Design review of the part shown in the three views and the two pictorial views. Dimensions are in mm from the part's minimum x, y and z. A direction names the side the tool comes from. Coordinates: 2 decimals unless noted, no trailing zeros. Loops run counter-clockwise (first coordinate to the right, second up) from the corner with the lowest first, then second, coordinate; pieces in that order, holes last. Notation, with made-up numbers: M 12.5,40 L 32.5,40 A28 ccw 32.5,79 Z; hole C 44,-20 d7. An arc over 180 degrees is marked long. Use one line per item in the form item = value.
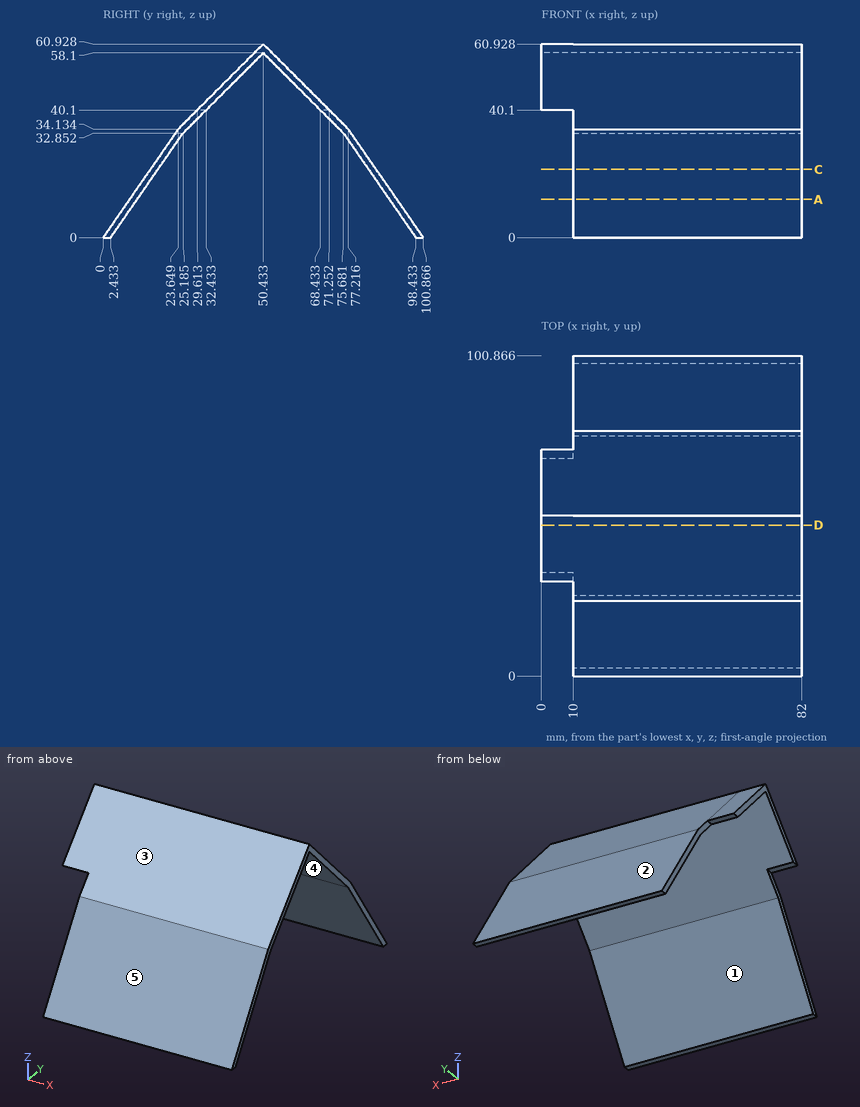
1. Insertion check: P1, Ø9.5, axis at y = 10.5, z = 22, coming from the -X side; P2, Ø1.4, axis at x = 6.5, y = 70, coming from the -Z side; P3, Ø2, axis at x = 51, z = 32, coming from the -Y side; P4, Ø3, axis at y = 83.5, z = 16.5, coming from the +X side. Each pin has a flat end and moves straight along its axis. Give the tip position at first contact, or say it passes through.
Response values:
P1 = 10
P2 = 40.1
P3 = 21.48
P4 = through
2. Add section A-A (z = 12). State the section outline as (x, y) points (1 decimal), then the cut area to 3 significant figures.
Response values:
outline = M 10,8.3 L 82,8.3 L 82,10.7 L 10,10.7 Z; M 10,90.1 L 82,90.1 L 82,92.6 L 10,92.6 Z
area = 350 mm^2
3. Machinability: for the marked faces 4 and 5, which of the approach directions +Z, -Z, +X, -X, +Y, -Y give a long, thin tool a straight path to every point of the face, cutting with its end or side? Answer none if there is none.
Response values:
face_4 = -Z, +X, -X
face_5 = +Z, +X, -X, -Y
4. Add section C-C (z = 21.5). State the section outline as (x, y) points.
Response values:
outline = M 10,14.9 L 82,14.9 L 82,17.32 L 10,17.32 Z; M 10,83.54 L 82,83.54 L 82,85.97 L 10,85.97 Z
5. Add section D-D (y = 47.5). State the section outline as (x, z) points (1 decimal).
Response values:
outline = M 0,55.2 L 82,55.2 L 82,58 L 0,58 Z
6. Wall thickness on line 1 along Y through (x, z) = (22.5, 42.5) (1 decimal); line 2 along Y through (x, z) = (22, 53) (1 decimal); line 3 along Z through (x, y) = (58.5, 41) (1 decimal): over which ranges is each line inside the solid? List them lowest first. Write a range as from..to.
Response values:
line_1 = 32..34.8, 66..68.9
line_2 = 42.5..45.3, 55.5..58.4
line_3 = 48.7..51.5
7. The part is to be moulded in two halves that separate along Y. For the marked faces 1, 2 and 3, say which applies: pulls with the +Y half, pulls with the -Y half, needs draft (parallel to the pull), parting line crosses it, or undercut.
Response values:
face_1 = undercut
face_2 = pulls with the +Y half
face_3 = pulls with the -Y half
